from build123d import *

# Parameters (mm, degrees)
SKETCH1_R           = 60
BOSS_EXTRUDE1_DEPTH = 3
SKETCH2_R           = 1.25
CUT_EXTRUDE1_DEPTH  = 4
SKETCH5_R           = 10
CUT_EXTRUDE2_DEPTH  = 4
SKETCH6_R           = 0.75
CUT_EXTRUDE3_DEPTH  = 4


with BuildPart() as part:
    # Sketch1 → Boss-Extrude1 (new body)
    with BuildSketch(Plane(origin=(0, 0, 0), x_dir=(1, 0, 0), z_dir=(0, 1, 0))):
        Circle(SKETCH1_R)
    extrude(amount=BOSS_EXTRUDE1_DEPTH)

    # Sketch2 → Cut-Extrude1 (cut, through all)
    with BuildSketch(Plane(origin=(0, 3, 0), x_dir=(1, 0, 0), z_dir=(0, 1, 0))):
        with Locations((-24.073102507, 45.644631202)):
            Circle(SKETCH2_R)
        with Locations((24.073102507, 45.644631202)):
            Circle(SKETCH2_R)
        with Locations((24.073102507, -45.644631202)):
            Circle(SKETCH2_R)
        with Locations((-24.073102507, -45.644631202)):
            Circle(SKETCH2_R)
    extrude(amount=-CUT_EXTRUDE1_DEPTH, mode=Mode.SUBTRACT)

    # Sketch5 → Cut-Extrude2 (cut, through all)
    with BuildSketch(Plane(origin=(0, 3, 0), x_dir=(1, 0, 0), z_dir=(0, 1, 0))):
        Circle(SKETCH5_R)
    extrude(amount=-CUT_EXTRUDE2_DEPTH, mode=Mode.SUBTRACT)

    # Sketch6 → Cut-Extrude3 (cut, through all)
    with BuildSketch(Plane(origin=(0, 3, 0), x_dir=(1, 0, 0), z_dir=(0, 1, 0))):
        with Locations((13.773714056, 48.12077632)):
            Circle(SKETCH6_R)
        with Locations((13.773714056, 16.62077632)):
            Circle(SKETCH6_R)
        with Locations((-13.773714056, 16.62077632)):
            Circle(SKETCH6_R)
        with Locations((-13.773714056, 48.12077632)):
            Circle(SKETCH6_R)
    extrude(amount=-CUT_EXTRUDE3_DEPTH, mode=Mode.SUBTRACT)


solid = part.part
Read the model definition and answer for the solid it produces. Units are mm, in the model's axes. Round coordinates to 2 decimals unless told otherwise and drop trailing zeros. Loops run counter-clockwise (first coordinate to the right, second up) from the corner with the lowest first, then second, coordinate; pieces in that order, holes last. Notation, with made-up numbers: (-5.75, 27) - (12.25, 27) arc R24 ccw to (12.25, 38) - close; hole circle Ø10 at (52, 40). An arc over 180 degrees is marked (long way). One line per question, with ' | ' between items. Start each with the question number.
Q1. For a pull along X with two mould halves and no side action, classify faces 1 (the cylindrical face through (-59.94, 1.48, -2.64)), 2 (the flat face through (12, 3, -1)), 3 (the cylindrical face through (-2.17, 1.52, 9.76)) as +X half, -X half, draft (parallel to the pull), parting line (faces both ways), or undercut.
Q2. Section D-D on x = -48 is taken. Give the vertices of the cut face in (y, z), plus the area to 3 significant figures.
Q3. Section C-C on y = 0.8 is taken. Count the separate pieces of the cut face and the enclosed holes in it, plus the area to 3 significant figures.
Q4. Section B-B on z = 0 is taken. Give the vertices of the cut face in (x, y).
Q5. Section A-A on x = 0 is taken. Give the vertices of the cut face in (y, z).
Q6. Find the intervals of material crossed by L1, parallel to X at y = 1.2, z = -45; L2, parallel to X at y = 0.3, z = 3.5; L3, parallel to X at y = 2.55, z = -4, in increasing order.
Established:
1) face 1: parting line | face 2: draft | face 3: undercut
2) outline: (0, -36) - (3, -36) - (3, 36) - (0, 36) - close | area: 216 mm²
3) separate pieces: 1 | enclosed holes: 9 | area: 11,000 mm²
4) outline: (-60, 0) - (-10, 0) - (-10, 3) - (-60, 3) - close; (10, 0) - (60, 0) - (60, 3) - (10, 3) - close
5) outline: (0, -60) - (3, -60) - (3, -10) - (0, -10) - close; (0, 10) - (3, 10) - (3, 60) - (0, 60) - close
6) L1: -39.69 to -25.14, -23 to 23, 25.14 to 39.69 | L2: -59.9 to -9.37, 9.37 to 59.9 | L3: -59.87 to -9.17, 9.17 to 59.87
